Source: three-view drawing plus pictorial views. Frame: mm from the lowest corner of the part. Give positions to 0.01 mm unless a question says otherwise; leave off trailing zeros. Order: outer loops, then holes, each group sorted by start corner. A loop starts at its lowest first (then second) coordinate and runs counter-clockwise, first axis right, second up. Notation, with made-up numbers: M -32.75,62 L 6.25,62 A22 ccw 6.25,79 Z; hole C 85,87.25 d3. An arc over 180 degrees is marked long. Use CSV: the item, a comma, the result in double quotes. Start each with the question number.
1. Pin query (flat end, axial travel): P1, Ø8, axis at x = 35.5, y = 11.5, coming from the +Z side; P2, Ø1, axis at x = 12.5, y = 28.5, coming from the -Z side. Return the tip coordinate at first contact, or that it passes through.
2. Section query A-A, the plane z = 8. Return the cut outline in (x, y).
3. Section query B-B, the plane y = 20.5. Return the cut outline in (x, z).
4. Section query D-D, the plane z = 40. Return the cut outline in (x, y).
5. Mould query, pull axis X, two halves, no side actions, for the marked faces 1, 2, 3 and 4. Classes: released by +X, released by -X, zero draft, split by the parting line, or undercut.
6. Section query C-C, the plane x = 41. Return the cut outline in (y, z).
7. Line query: line 1 along X through (y, z) = (41, 6); line 2 along Y through (x, z) = (34, 40). Output: solid intervals per line, ascending. Write a range as [from, to].
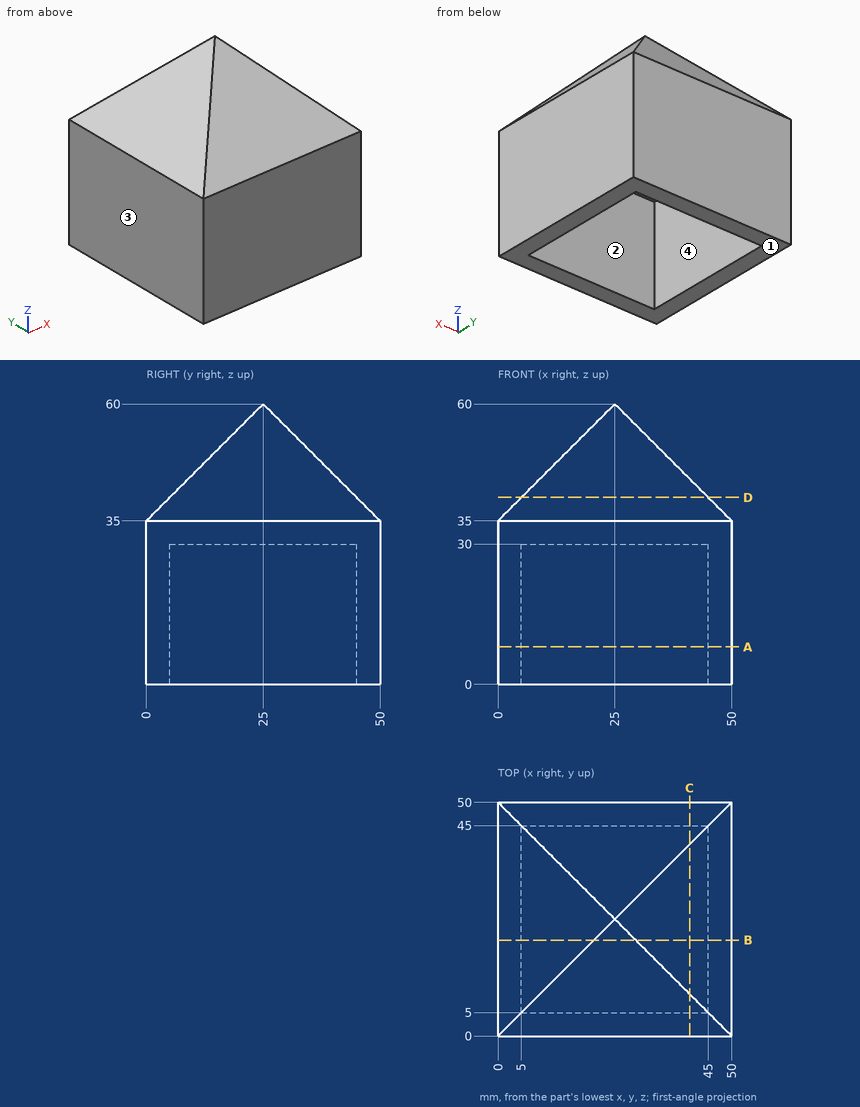
Result set:
1,P1,"z = 50.4"
1,P2,"z = 30"
2,outline,"M 0,0 L 50,0 L 50,50 L 0,50 Z; hole M 5,5 L 45,5 L 45,45 L 5,45 Z"
3,outline,"M 0,0 L 5,0 L 5,30 L 45,30 L 45,0 L 50,0 L 50,35 L 29.5,55.5 L 20.5,55.5 L 0,35 Z"
4,outline,"M 5,5 L 45,5 L 45,45 L 5,45 Z"
5,face 1,"zero draft"
5,face 2,"undercut"
5,face 3,"released by -X"
5,face 4,"undercut"
6,outline,"M 0,0 L 5,0 L 5,30 L 45,30 L 45,0 L 50,0 L 50,35 L 41,44 L 9,44 L 0,35 Z"
7,line 1,"[0, 5], [45, 50]"
7,line 2,"[5, 45]"
